Check sheet for the modelled part. Datum: model origin and axes. Units: mm. A direction names the side the tool comes from. Coordinates: 2 decimals unless noted, no trailing zeros. Loops run counter-clockwise (first coordinate to the right, second up) from the corner with the lowest first, then second, coordinate; pieces in that order, holes last. Notation, with made-up numbers: M -21.75,-28 L -3.75,-28 A33 ccw -3.75,3 Z; hole C -16,79.25 d2. An arc over 180 degrees is marked long. Return JSON: item names as keys, results as strings.
from build123d import *

# Parameters (mm, degrees)
F2_DEPTH = 25.4
F3_R     = 6.35
F4_DEPTH = 25.4
F5_DEPTH = 25.4


# Not quite as in the source:
# - a variable given as a bare number and used for a length is read in inches; the dataset says mm whatever the document's units were


with BuildPart() as f2:
    # F1 (on Top) → F2 (new body)
    with BuildSketch(Plane.XY):
        with BuildLine():
            ThreePointArc((-23.1655191958, -10.2824198201), (-10.4655191958, 2.4175801799), (-23.1655191958, 15.1175801799))
            Line((-23.1655191958, 15.1175801799), (-99.3655191958, 15.1175801799))
            ThreePointArc((-99.3655191958, 15.1175801799), (-112.0655191958, 2.4175801799), (-99.3655191958, -10.2824198201))
            Line((-99.3655191958, -10.2824198201), (-23.1655191958, -10.2824198201))
        make_face()
    extrude(amount=F2_DEPTH)

    # F3 (on face) → F4 (join)
    with BuildSketch(Plane.XY.offset(25.4)):
        with Locations((-99.3655191958, 2.4175801799)):
            Circle(F3_R)
    extrude(amount=F4_DEPTH)

    # F3 (on face) → F5 (cut)
    with BuildSketch(Plane.XY.offset(25.4)):
        with Locations((-23.1655191958, 2.4175801799)):
            Circle(F3_R)
    extrude(amount=-F5_DEPTH, mode=Mode.SUBTRACT)


solid = f2.part
1) Draft check along Y on faces 3 (the face through (-112.062, 2.697, 12.522)), 4 (the face through (-29.51, 2.7, 12.88)), 5 (the face through (-62, 3, 0)), 6 (the face through (-62, -10.282, 13)). Enter one of: +Y half, -Y half, draft (parallel to the pull), parting line (faces both ways), or undercut.
Answers:
{"face 3": "parting line", "face 4": "undercut", "face 5": "draft", "face 6": "-Y half"}
2) Scan lines: line 1 along Z through (x, y) = (-68.5, 12.5); line 2 along X through (y, z) = (1.5, 6); line 3 along X through (y, z) = (-2.5, 15). Record each from-to range of solid material in increasing order. Write a range as [from, to].
Answers:
{"line 1": "[0, 25.4]", "line 2": "[-112.03, -29.45], [-16.88, -10.5]", "line 3": "[-111.07, -27.18], [-19.15, -11.46]"}
3) Go/stop test with flat-tipped pins: pin 1 Ø8 at (y, z) = (-3.5, 26) entering from -X; pin 2 Ø10 at (y, z) = (12.5, 26.5) entering from -X; pin 3 Ø12.5 at (x, y) = (-54.5, -0.5) entering from +Z. Record where each tip stops, or that it passes through.
Answers:
{"pin 1": "x = -111.91", "pin 2": "x = -110.95", "pin 3": "z = 25.4"}
4) Section check B-B on x = -21.5. Record the cut outline in (y, z).
Answers:
{"outline": "M -10.17,0 L -3.71,0 L -3.71,25.4 L -10.17,25.4 Z; M 8.55,0 L 15.01,0 L 15.01,25.4 L 8.55,25.4 Z"}
5) Section check D-D on x = -102. Record the cut outline in (y, z).
Answers:
{"outline": "M -10.01,0 L 14.84,0 L 14.84,25.4 L 8.2,25.4 L 8.2,50.8 L -3.36,50.8 L -3.36,25.4 L -10.01,25.4 Z"}
6) Section check A-A on y = 3.5. Record the cut outline in (x, z).
Answers:
{"outline": "M -112.02,0 L -29.42,0 L -29.42,25.4 L -93.11,25.4 L -93.11,50.8 L -105.62,50.8 L -105.62,25.4 L -112.02,25.4 Z; M -16.91,0 L -10.51,0 L -10.51,25.4 L -16.91,25.4 Z"}
7) Section check C-C on z = 7. Record the cut outline in (x, y), then the cut area to 3 significant figures.
Answers:
{"outline": "M -99.37,-10.28 L -23.17,-10.28 A12.7 ccw -23.17,15.12 L -99.37,15.12 A12.7 ccw Z; hole C -23.17,2.42 d12.7", "area": "2,320 mm²"}
8) Set-up check for faces 1 (the face through (-93.3, 4.3, 37.9)), 2 (the face through (-10.47, 2.14, 12.52)): record each of +Z, -Z, +X, -X, +Y, -Y from which the full face is reachable in a straight line by a thin tool's end or side.
Answers:
{"face 1": "+Z", "face 2": "+Z, -Z, +X"}
